```python
from build123d import *

# Parameters (mm, degrees)
SKETCH1_R      = 10
SKETCH1_W      = 50
SKETCH1_H      = 10
EXTRUDE1_DEPTH = 10


with BuildPart() as part:
    # Sketch1 → Extrude1 (new body)
    # profile 1 of 2: a face of its own
    with BuildSketch(Plane.XY):
        with BuildLine():
            Line((-14.889688552, 19.935237795), (-14.889688552, 4.935237795))
            Line((-14.889688552, 4.935237795), (15.110311448, 4.935237795))
            Line((15.110311448, 4.935237795), (15.110311448, 19.935237795))
            ThreePointArc((15.110311448, 19.935237795), (0.110311448, 34.935237795), (-14.889688552, 19.935237795))
        make_face()
        with Locations((0.110311448, 19.935237795)):
            Circle(SKETCH1_R, mode=Mode.SUBTRACT)
    # profile 2 of 2: a face of its own
    with BuildSketch(Plane.XY):
        with Locations((0.110311448, -0.064762205)):
            Rectangle(SKETCH1_W, SKETCH1_H)
    extrude(amount=EXTRUDE1_DEPTH)


solid = part.part
```
Verification items for the finished model (mm, model axes). A direction names the side the tool comes from. Round coordinates to 2 decimals unless told otherwise and drop trailing zeros. Loops run counter-clockwise (first coordinate to the right, second up) from the corner with the lowest first, then second, coordinate; pieces in that order, holes last. Notation, with made-up numbers: (-29.5, 14.25) -> (-23.5, 14.25) arc R29 cw to (-23.5, 43.25) -> close; hole circle Ø7 at (-22, 87.25). An arc over 180 degrees is marked (long way). Answer as a JSON object with one key per item and string values.
Q1. Section check D-D (x = 17). Record the boundary of the cut face in (y, z).
Data:
{"outline": "(-5.06, 0) -> (4.94, 0) -> (4.94, 10) -> (-5.06, 10) -> close"}
Q2. Access from +Z, -Z, +X, -X, +Y, -Y to the whole of each face (thin tool, end or side, straight path). Record for faces 5 (the flat face through (0, 6, 10)), 6 (the flat face through (15.11, 12, 5)), 7 (the flat face through (-14.89, 13, 5)).
Data:
{"face 5": "+Z, +X, -X, +Y, -Y", "face 6": "+Z, -Z, +X, +Y", "face 7": "+Z, -Z, -X, +Y"}
Q3. Section check C-C (y = 18). Record the boundary of the cut face in (x, z).
Data:
{"outline": "(-14.89, 0) -> (-9.7, 0) -> (-9.7, 10) -> (-14.89, 10) -> close; (9.92, 0) -> (15.11, 0) -> (15.11, 10) -> (9.92, 10) -> close"}
Q4. Section check B-B (x = 2). Record the boundary of the cut face in (y, z), then the cut area to 3 significant figures.
Data:
{"outline": "(-5.06, 0) -> (10.12, 0) -> (10.12, 10) -> (-5.06, 10) -> close; (29.76, 0) -> (34.82, 0) -> (34.82, 10) -> (29.76, 10) -> close", "area": "202 mm2"}
Q5. Scan lines: line 1 (Y direction, x = 0.5, z = 3.75); line 2 (Y direction, x = 16, z = 4); line 3 (X direction, y = 19.5, z = 3). Record each from-to range of solid material in increasing order. Write a range as from..to.
Data:
{"line 1": "y = -5.06..9.94, 29.93..34.93", "line 2": "y = -5.06..4.94", "line 3": "x = -14.89..-9.88, 10.1..15.11"}
Q6. Draft check along Y on faces 1 (the flat face through (25.11, 0, 5)), 2 (the flat face through (0, -5.065, 5)), 3 (the cylindrical face through (-2.057, 10.173, 4.93)), 4 (the flat face through (20, 4.935, 5)). Enter one of: pulls with the +Y half, pulls with the -Y half, needs draft (parallel to the pull), parting line crosses it, or undercut.
Data:
{"face 1": "needs draft", "face 2": "pulls with the -Y half", "face 3": "undercut", "face 4": "pulls with the +Y half"}
Q7. Section check A-A (z = 8.5). Record the boundary of the cut face in (x, y).
Data:
{"outline": "(-24.89, -5.06) -> (25.11, -5.06) -> (25.11, 4.94) -> (15.11, 4.94) -> (15.11, 19.94) arc R15 ccw to (-14.89, 19.94) -> (-14.89, 4.94) -> (-24.89, 4.94) -> close; hole circle Ø20 at (0.11, 19.94)"}
Q8. Go/stop test with flat-tipped pins: P1, Ø1, axis at y = 14.5, z = 5, coming from the -X side; P2, Ø12, axis at x = -5.5, y = 11, coming from the -Z side; P3, Ø1.5, axis at x = -7, z = 3.5, coming from the +Y side; P4, Ø6, axis at y = 28.5, z = 2.5, coming from the +X side. Record where each tip stops, or that it passes through.
Data:
{"P1": "stops at x = -14.89", "P2": "stops at z = 0", "P3": "stops at y = 33.52", "P4": "stops at x = 14.04"}
